Input: part model. Units: mm. Frame: model coordinates. A direction names the side the tool comes from. Give positions to 0.01 mm unless a question says otherwise; leave off trailing zeros. Write each loop counter-clockwise with the first axis right and the second up, starting at its lowest first coordinate (ties: lowest second). Pieces come first, ordered by that corner, then holes.
```python
from build123d import *

# Parameters (mm, degrees)
SZKIC1_W                    = 77.5
SZKIC1_H                    = 42.8
SZKIC1_R                    = 1.6
DODANIE_WYCI_GNI_CIE1_DEPTH = 1.7
SZKIC2_W                    = 60
SZKIC2_H                    = 42.8
DODANIE_WYCI_GNI_CIE2_DEPTH = 4
DODANIE_WYCI_GNI_CIE3_DEPTH = 3
SZKIC4_W                    = 3.5
SZKIC4_H                    = 35.7
DODANIE_WYCI_GNI_CIE4_DEPTH = 8.5
SZKIC5_W                    = 20.589223083
SZKIC5_H                    = 59.264583933
SZKIC5_W_2                  = 0.5
SZKIC5_H_2                  = 0.5
WYTNIJ_WYCI_GNI_CIE1_DEPTH  = 7


with BuildPart() as part:
    # Szkic1 → Dodanie-wyciągnięcie1 (new body)
    with BuildSketch(Plane(origin=(0, 0, 0), x_dir=(1, 0, 0), z_dir=(0, 1, 0))):
        Rectangle(SZKIC1_W, SZKIC1_H)
        with Locations((-35.75, 18.4)):
            Circle(SZKIC1_R, mode=Mode.SUBTRACT)
        with Locations((31.55, 18.4)):
            Circle(SZKIC1_R, mode=Mode.SUBTRACT)
        with Locations((31.55, -18.3)):
            Circle(SZKIC1_R, mode=Mode.SUBTRACT)
        with Locations((-35.75, -18.3)):
            Circle(SZKIC1_R, mode=Mode.SUBTRACT)
    extrude(amount=DODANIE_WYCI_GNI_CIE1_DEPTH)

    # Szkic2 → Dodanie-wyciągnięcie2 (add)
    with BuildSketch(Plane(origin=(0, 1.7, 0), x_dir=(1, 0, 0), z_dir=(0, 1, 0))):
        with Locations((-1.75, 0)):
            Rectangle(SZKIC2_W, SZKIC2_H)
    extrude(amount=DODANIE_WYCI_GNI_CIE2_DEPTH)

    # Szkic3 → Dodanie-wyciągnięcie3 (add)
    with BuildSketch(Plane.XZ):
        Polygon((4.05, 21.4), (4.05, 4.5), (-20.45, 4.5), (-20.45, 9.5), (-22.35, 12.4), (-22.35, 21.4), align=None)
    extrude(amount=DODANIE_WYCI_GNI_CIE3_DEPTH)

    # Szkic4 → Dodanie-wyciągnięcie4 (add)
    with BuildSketch(Plane.XZ):
        with Locations((36.3, -0.05)):
            Rectangle(SZKIC4_W, SZKIC4_H)
    extrude(amount=DODANIE_WYCI_GNI_CIE4_DEPTH)

    # Szkic5 → Wytnij-wyciągnięcie1 (cut)
    with BuildSketch(Plane.XZ.offset(8.5)):
        with Locations((39.347598483, -1.41955971)):
            Rectangle(SZKIC5_W, SZKIC5_H)
        with Locations((36.3, 16.525)):
            Rectangle(SZKIC5_W_2, SZKIC5_H_2, mode=Mode.SUBTRACT)
        with Locations((36.3, 13.975)):
            Rectangle(SZKIC5_W_2, SZKIC5_H_2, mode=Mode.SUBTRACT)
        with Locations((36.3, 11.425)):
            Rectangle(SZKIC5_W_2, SZKIC5_H_2, mode=Mode.SUBTRACT)
        with Locations((36.3, 8.875)):
            Rectangle(SZKIC5_W_2, SZKIC5_H_2, mode=Mode.SUBTRACT)
        with Locations((36.3, 6.325)):
            Rectangle(SZKIC5_W_2, SZKIC5_H_2, mode=Mode.SUBTRACT)
        with Locations((36.3, 3.775)):
            Rectangle(SZKIC5_W_2, SZKIC5_H_2, mode=Mode.SUBTRACT)
        with Locations((36.3, 1.225)):
            Rectangle(SZKIC5_W_2, SZKIC5_H_2, mode=Mode.SUBTRACT)
        with Locations((36.3, -1.325)):
            Rectangle(SZKIC5_W_2, SZKIC5_H_2, mode=Mode.SUBTRACT)
        with Locations((36.3, -3.875)):
            Rectangle(SZKIC5_W_2, SZKIC5_H_2, mode=Mode.SUBTRACT)
        with Locations((36.3, -6.425)):
            Rectangle(SZKIC5_W_2, SZKIC5_H_2, mode=Mode.SUBTRACT)
        with Locations((36.3, -8.975)):
            Rectangle(SZKIC5_W_2, SZKIC5_H_2, mode=Mode.SUBTRACT)
        with Locations((36.3, -11.525)):
            Rectangle(SZKIC5_W_2, SZKIC5_H_2, mode=Mode.SUBTRACT)
        with Locations((36.3, -14.075)):
            Rectangle(SZKIC5_W_2, SZKIC5_H_2, mode=Mode.SUBTRACT)
        with Locations((36.3, -16.625)):
            Rectangle(SZKIC5_W_2, SZKIC5_H_2, mode=Mode.SUBTRACT)
    extrude(amount=-WYTNIJ_WYCI_GNI_CIE1_DEPTH, mode=Mode.SUBTRACT)


solid = part.part
```
Q1. Access query for faces 5 (the flat face through (-21.387, -1.479, 10.93)), 6 (the flat face through (38.75, 1, 0)), 7 (the flat face through (33, 1.7, 0)), 8 (the flat face through (36, -1, -17.9)), 9 (the flat face through (36, -1, 17.8)). Directions: +Z, -Z, +X, -X, +Y, -Y. A direction counts if a zero-diameter tool reaches every point of the face in a straight line with its end or side. Return the directions, or none.
Q2. Section A-A, the plane x = -35.75. Return the cut outline in (y, z).
Q3. Mould query, pull axis X, two halves, no side actions, for faces 1 (the cylindrical face through (-36.1, 0.84, -16.84)), 2 (the flat face through (34.55, -1, 0)), 3 (the flat face through (28.25, 4, 0)), 4 (the flat face through (-31.75, 4, 0)). Classes: +X half, -X half, draft (parallel to the pull), parting line (faces both ways), or undercut.
Q4. Section D-D, the plane x = -11.5. Return the cut outline in (y, z), then the cut area to 3 significant figures.
Q5. Pin query (flat end, axial travel): pin 1 (1.6 mm diameter, centred on x = 35.5, y = -1, fed in from -Z); pin 2 (8 mm diameter, centred on y = -7, z = -14.5, fed in from +X); pin 3 (2 mm diameter, centred on x = 0, y = -3, fed in from -Z). Return the tip coordinate at first contact, or that it passes through.
Q6. Material intervals for line 1 along X through (y, z) = (0.9, -18.4); line 2 along Z through (x, y) = (31.55, 1.2); line 3 along Y through (x, z) = (8.5, -16), sorted ascending.
Q7. Section C-C, the plane z = -13. Return the cut outline in (x, y).
Q8. Section B-B, the plane y = -6.25. Give the number of separate pieces and of enclosed holes in the cut face, then the cut area to 3 significant figures.
Solutions:
1. face 5: -Z, -X, -Y
1. face 6: +Z, -Z, +X, +Y, -Y
1. face 7: +Z, -Z, +X, +Y
1. face 8: -Z, +X, -X, -Y
1. face 9: +Z, +X, -Y
2. outline: (0, -21.4) - (1.7, -21.4) - (1.7, -20) - (0, -20) - close; (0, -16.8) - (1.7, -16.8) - (1.7, 16.7) - (0, 16.7) - close; (0, 19.9) - (1.7, 19.9) - (1.7, 21.4) - (0, 21.4) - close
3. face 1: undercut
3. face 2: undercut
3. face 3: +X half
3. face 4: -X half
4. outline: (-3, 4.5) - (0, 4.5) - (0, -21.4) - (5.7, -21.4) - (5.7, 21.4) - (-3, 21.4) - close
4. area: 295 mm2
5. pin 1: stops at z = -17.9
5. pin 2: stops at x = 36.55
5. pin 3: stops at z = 4.5
6. line 1: x = -38.75 to -37.35, -34.15 to 29.95, 33.15 to 38.75
6. line 2: z = -21.4 to -20, -16.8 to 16.7, 19.9 to 21.4
6. line 3: y = 0 to 5.7
7. outline: (-38.75, 0) - (34.55, 0) - (34.55, -1.5) - (38.05, -1.5) - (38.05, 0) - (38.75, 0) - (38.75, 1.7) - (28.25, 1.7) - (28.25, 5.7) - (-31.75, 5.7) - (-31.75, 1.7) - (-38.75, 1.7) - close
8. separate pieces: 14
8. enclosed holes: 0
8. area: 3.50 mm2
